```python
from build123d import *

# Parameters (mm, degrees)
SKETCH1_W           = 40
SKETCH1_H           = 20
BOX_DEPTH           = 20
SKETCH10_R          = 6
SIDE_CUT_DEPTH      = 4
CUT_EXTRUDE10_DEPTH = 20
CUT_EXTRUDE11_DEPTH = 4
CUT_EXTRUDE12_DEPTH = 20


with BuildPart() as part:
    # Sketch1 → Box (new body)
    with BuildSketch(Plane.XY):
        with Locations((-4.957264957, 0)):
            Rectangle(SKETCH1_W, SKETCH1_H)
    extrude(amount=BOX_DEPTH)

    # Sketch10 → Side Cut (cut)
    with BuildSketch(Plane.XY.offset(20)):
        with Locations((5.042735043, 0)):
            Circle(SKETCH10_R)
    extrude(amount=-SIDE_CUT_DEPTH, mode=Mode.SUBTRACT)

    # Sketch11 → Cut-Extrude10 (cut)
    with BuildSketch(Plane.XY.offset(20)):
        with BuildLine():
            ThreePointArc((7.042735043, 0), (6.456948605, 1.414213562), (5.042735043, 2))
            Line((5.042735043, 2), (5.042735043, -2))
            ThreePointArc((5.042735043, -2), (6.456948605, -1.414213562), (7.042735043, 0))
        make_face()
        with BuildLine():
            Line((5.042735043, -2), (5.042735043, 2))
            ThreePointArc((5.042735043, 2), (3.042735043, 0), (5.042735043, -2))
        make_face()
    extrude(amount=-CUT_EXTRUDE10_DEPTH, mode=Mode.SUBTRACT)

    # Sketch12 → Cut-Extrude11 (cut)
    with BuildSketch(Plane(origin=(0, 10, 0), x_dir=(1, 0, 0), z_dir=(0, 1, 0))):
        with BuildLine():
            ThreePointArc((-8.957264957, -10), (-14.957264957, -4), (-20.957264957, -10))
            Line((-20.957264957, -10), (-8.957264957, -10))
        make_face()
        with BuildLine():
            Line((-8.957264957, -10), (-20.957264957, -10))
            ThreePointArc((-20.957264957, -10), (-14.957264957, -16), (-8.957264957, -10))
        make_face()
    extrude(amount=-CUT_EXTRUDE11_DEPTH, mode=Mode.SUBTRACT)

    # Sketch13 → Cut-Extrude12 (cut)
    with BuildSketch(Plane(origin=(0, 10, 0), x_dir=(1, 0, 0), z_dir=(0, 1, 0))):
        with BuildLine():
            ThreePointArc((-12.957264957, -10), (-13.543051395, -8.585786438), (-14.957264957, -8))
            Line((-14.957264957, -8), (-14.957264957, -12))
            ThreePointArc((-14.957264957, -12), (-13.543051395, -11.414213562), (-12.957264957, -10))
        make_face()
        with BuildLine():
            Line((-14.957264957, -12), (-14.957264957, -8))
            ThreePointArc((-14.957264957, -8), (-16.957264957, -10), (-14.957264957, -12))
        make_face()
    extrude(amount=-CUT_EXTRUDE12_DEPTH, mode=Mode.SUBTRACT)


solid = part.part
```
The model under review builds one solid part; all positions refer to its coordinate system, in mm. A direction names the side the tool comes from. Coordinates: 2 decimals unless noted, no trailing zeros. Write each loop counter-clockwise with the first axis right and the second up, starting at its lowest first coordinate (ties: lowest second). Pieces come first, ordered by that corner, then holes.
1) We need section A-A on y = -1.5. State the section outline as (x, z) points.
2) Clearance check with flat-ended pins moving along their axes: pin 1 Ø8 at (x, y) = (-11.5, 6.5) entering from -Z; pin 2 Ø3.5 at (x, y) = (2, -1) entering from +Z; pin 3 Ø6 at (x, z) = (-15.5, 8) entering from +Y. State where each tip first meets the part, or that it passes through.
3) We need section C-C on x = -11. State the section outline as (y, z) points, then the cut area to 3 significant figures.
4) We need section D-D on y = 7.75. State the section outline as (x, z) points, then the cut area to 3 significant figures.
5) We need section B-B on z = 3.5. State the section outline as (x, y) points.
6) To check wall thickness, follow probe 1 along Z at (x, y) = (7, 3.5); probe 2 along X at (y, z) = (2.5, 11.5); probe 3 along Z at (x, y) = (-14, -4.25). State the ranges of each line that lie inside material, in increasing order.
7) The part is to be moulded in two halves that separate along X. For faces 4 (the face through (-5, 0, 0)), 5 (the face through (10.585, -2.298, 18.028)), 6 (the face through (15.043, 0, 10)), 7 (the face through (-24.957, 0, 10)), say which applies: pulls with the +X half, pulls with the -X half, needs draft (parallel to the pull), parting line crosses it, or undercut.
8) Machinability: for faces 1 (the face through (-12, 6, 10)), 2 (the face through (-5, -10, 10)), 3 (the face through (8, 0, 16)), which of the approach directions +Z, -Z, +X, -X, +Y, -Y give a long, thin tool a straight path to every point of the face, cutting with its end or side? Answer none if there is none.
Answer list:
1. outline: (-24.96, 0) - (3.72, 0) - (3.72, 16) - (-0.77, 16) - (-0.77, 20) - (-24.96, 20) - close; (6.37, 0) - (15.04, 0) - (15.04, 20) - (10.85, 20) - (10.85, 16) - (6.37, 16) - close; hole circle Ø4 at (-14.96, 10)
2. pin 1: stops at z = 0
2. pin 2: stops at z = 16
2. pin 3: stops at y = 6
3. outline: (-10, 0) - (10, 0) - (10, 5.49) - (6, 5.49) - (6, 14.51) - (10, 14.51) - (10, 20) - (-10, 20) - close
3. area: 364 mm2
4. outline: (-24.96, 0) - (15.04, 0) - (15.04, 20) - (-24.96, 20) - close; hole circle Ø12 at (-14.96, 10)
4. area: 687 mm2
5. outline: (-24.96, -10) - (15.04, -10) - (15.04, 10) - (-24.96, 10) - close; hole circle Ø4 at (5.04, 0)
6. probe 1: z = 0 to 16
6. probe 2: x = -24.96 to -16.28, -13.63 to 15.04
6. probe 3: z = 0 to 8.24, 11.76 to 20
7. face 4: needs draft
7. face 5: undercut
7. face 6: pulls with the +X half
7. face 7: pulls with the -X half
8. face 1: +Y
8. face 2: +Z, -Z, +X, -X, -Y
8. face 3: +Z
